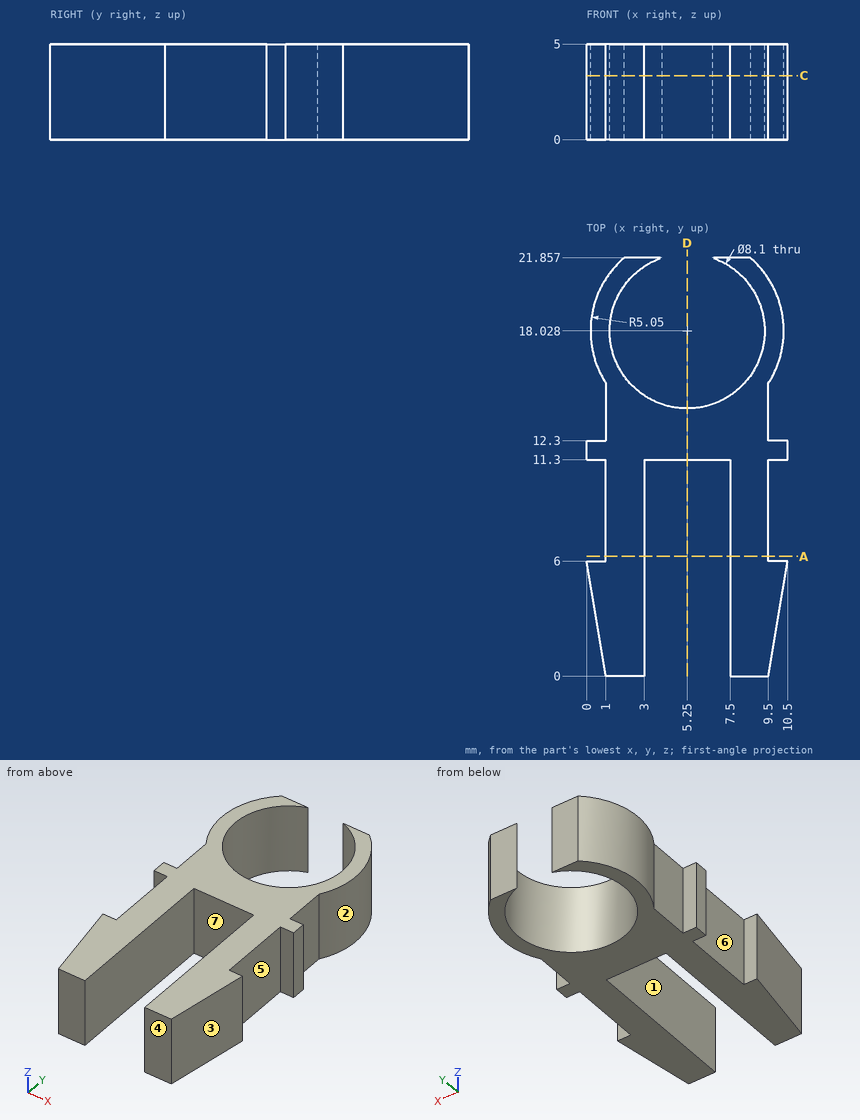
Could you check a few things on this drawing? It's one solid part, dimensions in mm from its lowest x, y, z. A direction names the side the tool comes from. Round coordinates to 2 decimals unless told otherwise and drop trailing zeros. Loops run counter-clockwise (first coordinate to the right, second up) from the corner with the lowest first, then second, coordinate; pieces in that order, holes last. Notation, with made-up numbers: M -37.5,38.25 L -32.5,38.25 A19 ccw -32.5,75.25 Z; hole C -17.5,89 d1. An arc over 180 degrees is marked long. Write item = value, one per line. Start each with the question number.
(1) Which directions (+Z, -Z, +X, -X, +Y, -Y) give clear straight access to the entire face, cutting with the end or side of a thin tool? Please do the marked faces 4, 5, 6 and 7.
(2) Suppose I cut it at A-A on y = 6.25. Write out the boundary of the cut face in (x, z), plus the area to 3 significant figures.
(3) I'm going to push flat-ended pins straight in: P1, Ø2, axis at y = 17, z = 4, coming from the -X side; P2, Ø0.9, axis at y = 14, z = 3, coming from the -X side; P3, Ø1.3, axis at x = 6, z = 2, coming from the -Y side. Where does each tip first touch, or does it pass through?
(4) Suppose I cut it at C-C on z = 3.35. Write out the boundary of the cut face in (x, y).
(5) I need wall thicknesses on line 1 along X through (y, z) = (8.25, 4.85); line 2 along Y through (x, z) = (5.25, 2.5); line 3 along Y through (x, z) = (8, 3.5) (1 decimal). Which ranges of each line are inside material? Lowest first, please.
(6) If we mould it in two halves opening along Y, with no side actions, what happens to the marked faces 1, 2 and 3? For each: released by +Y, released by -Y, zero draft, split by the parting line, or undercut.
(7) Suppose I cut it at D-D on x = 5.25. Write out the boundary of the cut face in (y, z), plus the area to 3 significant figures.
Answer block:
q1.face_4 = +Z, -Z, +X, -X, -Y
q1.face_5 = +Z, -Z, +X
q1.face_6 = +Z, -Z, -X
q1.face_7 = +Z, -Z, -Y
q2.outline = M 1,0 L 3,0 L 3,5 L 1,5 Z; M 7.5,0 L 9.5,0 L 9.5,5 L 7.5,5 Z
q2.area = 20.0 mm²
q3.P1 = 0.2
q3.P2 = 1
q3.P3 = 11.3
q4.outline = M 0,6 L 1,0 L 3,0 L 3,11.3 L 7.5,11.3 L 7.5,0 L 9.5,0 L 10.5,6 L 9.5,6 L 9.5,11.3 L 10.5,11.3 L 10.5,12.3 L 9.5,12.3 L 9.5,15.3 A5.05 ccw 8.54,21.86 L 6.57,21.86 A4.05 cw long 3.93,21.86 L 1.96,21.86 A5.05 ccw 1,15.3 L 1,12.3 L 0,12.3 L 0,11.3 L 1,11.3 L 1,6 Z
q5.line_1 = 1 to 3, 7.5 to 9.5
q5.line_2 = 11.3 to 13.98
q5.line_3 = 0 to 15.1, 21 to 21.9
q6.face_1 = zero draft
q6.face_2 = undercut
q6.face_3 = released by -Y
q7.outline = M 11.3,0 L 13.98,0 L 13.98,5 L 11.3,5 Z
q7.area = 13.4 mm²
